Model file for the job. Use its own axes, mm. A direction names the side the tool comes from. Give positions to 0.01 mm unless a question says otherwise; leave off trailing zeros. Write each loop counter-clockwise with the first axis right and the second up, starting at its lowest first coordinate (ties: lowest second). Pieces come first, ordered by that corner, then holes.
```python
from build123d import *

# Parameters (mm, degrees)
SKETCH1_R            = 33.5
BOSS_EXTRUDE3_DEPTH  = 16.5
SKETCH2_W            = 20
SKETCH2_H            = 39
BOSS_EXTRUDE4_DEPTH  = 34.758
SKETCH3_R            = 10
SKETCH3_R_2          = 6.5
BOSS_EXTRUDE5_DEPTH  = 2
SKETCH3_3_R          = 6.5
BOSS_EXTRUDE6_DEPTH  = 3
SKETCH3_4_R          = 2.85
BOSS_EXTRUDE7_DEPTH  = 7.3
SKETCH5_W            = 11
SKETCH5_H            = 3.5
SKETCH5_W_2          = 3.5
SKETCH5_H_2          = 8
BOSS_EXTRUDE8_DEPTH  = 34.758
SKETCH6_W            = 11
SKETCH6_H            = 8
BOSS_EXTRUDE9_DEPTH  = 3.5
SKETCH7_R            = 2.5
BOSS_EXTRUDE10_DEPTH = 6
FILLET1_R            = 3.5
FILLET2_R            = 3.5
FILLET3_R            = 3.5
FILLET4_R            = 3.5
SKETCH9_W            = 3.5
SKETCH9_H            = 20
BOSS_EXTRUDE11_DEPTH = 30.867
SKETCH9_3_W          = 3.5
SKETCH9_3_H          = 11
BOSS_EXTRUDE12_DEPTH = 27
CUT_EXTRUDE1_DEPTH   = 88.052447203
BOSS_EXTRUDE13_START = 3
SKETCH10_3_R         = 10
BOSS_EXTRUDE13_DEPTH = 3
SKETCH10_4_R         = 5
SKETCH10_4_R_2       = 3
BOSS_EXTRUDE14_DEPTH = 4.5
CUT_EXTRUDE4_START   = -18.5
SKETCH10_7_R         = 1.5
CUT_EXTRUDE4_DEPTH   = 34.5
CIRPATTERN3_COUNT    = 4
SKETCH11_R           = 1.5
CUT_EXTRUDE6_DEPTH   = 86.054856205
SKETCH13_R           = 2.7
CUT_EXTRUDE10_DEPTH  = 15.5
CUT_EXTRUDE11_DEPTH  = 3.5
CIRPATTERN4_COUNT    = 4
SKETCH14_3_R         = 1.25
CUT_EXTRUDE12_DEPTH  = 3.5


with BuildPart() as part:
    # Sketch1 → Boss-Extrude3 (new body)
    with BuildSketch(Plane.XY):
        Circle(SKETCH1_R)
    extrude(amount=BOSS_EXTRUDE3_DEPTH)

    # Sketch2 → Boss-Extrude4 (add)
    with BuildSketch(Plane.XY.offset(16.5)):
        Rectangle(SKETCH2_W, SKETCH2_H)
    extrude(amount=BOSS_EXTRUDE4_DEPTH)

    # Sketch3 → Boss-Extrude5 (add)
    with BuildSketch(Plane(origin=(0, 19.5, 0), x_dir=(1, 0, 0), z_dir=(0, 1, 0))):
        with Locations(Location((0, -41.258, 0), (0, 0, 270))):
            Circle(SKETCH3_R)
        with Locations(Location((0, -41.258, 0), (0, 0, 270))):
            Circle(SKETCH3_R_2, mode=Mode.SUBTRACT)
    extrude(amount=BOSS_EXTRUDE5_DEPTH)

    # Sketch3<3> → Boss-Extrude6 (add)
    with BuildSketch(Plane(origin=(0, 19.5, 0), x_dir=(1, 0, 0), z_dir=(0, 1, 0))):
        with Locations(Location((0, -41.258, 0), (0, 0, 270))):
            Circle(SKETCH3_3_R)
    extrude(amount=BOSS_EXTRUDE6_DEPTH)

    # Sketch3<4> → Boss-Extrude7 (add)
    with BuildSketch(Plane(origin=(0, 19.5, 0), x_dir=(1, 0, 0), z_dir=(0, 1, 0))):
        with Locations(Location((0, -41.258, 0), (0, 0, 270))):
            Circle(SKETCH3_4_R)
    extrude(amount=BOSS_EXTRUDE7_DEPTH)

    # Sketch5 → Boss-Extrude8 (add)
    with BuildSketch(Plane.XY.offset(51.258)):
        with Locations((0, -21.25)):
            Rectangle(SKETCH5_W, SKETCH5_H)
        with Locations((11.75, 7.5)):
            Rectangle(SKETCH5_W_2, SKETCH5_H_2)
        with Locations((-11.75, 7.5)):
            Rectangle(SKETCH5_W_2, SKETCH5_H_2)
    extrude(amount=-BOSS_EXTRUDE8_DEPTH)

    # Sketch6 → Boss-Extrude9 (add)
    with BuildSketch(Plane.XY.offset(51.258)):
        with Locations((0, 7.5)):
            Rectangle(SKETCH6_W, SKETCH6_H)
        Polygon((10, 11.5), (5.5, 11.5), (5.5, 3.5), (10, 3.5), (13.5, 3.5), (13.5, 11.5), align=None)
        Polygon((5.5, 3.5), (-5.5, 3.5), (-5.5, -19.5), (-5.5, -23), (5.5, -23), (5.5, -19.5), align=None)
        Polygon((-10, 11.5), (-13.5, 11.5), (-13.5, 3.5), (-10, 3.5), (-5.5, 3.5), (-5.5, 11.5), align=None)
    extrude(amount=BOSS_EXTRUDE9_DEPTH)

    # Sketch7 → Boss-Extrude10 (add)
    with BuildSketch(Plane.XZ.offset(23)):
        with Locations(Location((0, 41.258, 0), (0, 0, 270))):
            Circle(SKETCH7_R)
    extrude(amount=BOSS_EXTRUDE10_DEPTH)

    # Fillet1
    fillet1_edges = [part.edges().sort_by_distance(p)[0] for p in [
        (-13.5, 7.5, 54.758),
        (13.5, 7.5, 54.758),
    ]]
    fillet(fillet1_edges, radius=FILLET1_R)

    # Fillet2
    fillet2_edges = [part.edges().sort_by_distance(p)[0] for p in [
        (0, -23, 54.758),
    ]]
    fillet(fillet2_edges, radius=FILLET2_R)

    # Fillet3
    fillet3_edges = [part.edges().sort_by_distance(p)[0] for p in [
        (13.5, 7.5, 16.5),
    ]]
    fillet(fillet3_edges, radius=FILLET3_R)

    # Fillet4
    fillet4_edges = [part.edges().sort_by_distance(p)[0] for p in [
        (-13.5, 7.5, 16.5),
    ]]
    fillet(fillet4_edges, radius=FILLET4_R)

    # Sketch9 → Boss-Extrude11 (add)
    with BuildSketch(Plane(origin=(0, 0, 0), x_dir=(-1, 0, 0), z_dir=(0, 0, -1))):
        with Locations((27.05, 0)):
            Rectangle(SKETCH9_W, SKETCH9_H)
    extrude(amount=BOSS_EXTRUDE11_DEPTH)

    # Sketch9<3> → Boss-Extrude12 (add)
    with BuildSketch(Plane(origin=(0, 0, 0), x_dir=(-1, 0, 0), z_dir=(0, 0, -1))):
        with Locations((-27.25, 0)):
            Rectangle(SKETCH9_3_W, SKETCH9_3_H)
    extrude(amount=BOSS_EXTRUDE12_DEPTH)

    # Sketch10 → Cut-Extrude1 (cut, through all)
    with BuildSketch(Plane(origin=(-25.3, 0, 0), x_dir=(0, 0, -1), z_dir=(1, 0, 0))):
        with BuildLine():
            ThreePointArc((20.867, 10), (27.938067812, 7.071067812), (30.867, 0))
            Line((30.867, 0), (30.867, 10))
            Line((30.867, 10), (20.867, 10))
        make_face()
        with BuildLine():
            Line((30.867, -10), (30.867, 0))
            ThreePointArc((30.867, 0), (27.938067812, -7.071067812), (20.867, -10))
            Line((20.867, -10), (30.867, -10))
        make_face()
    extrude(amount=-CUT_EXTRUDE1_DEPTH, mode=Mode.SUBTRACT)

    # Sketch10<3> → Boss-Extrude13 (add)
    with BuildSketch(Plane(origin=(-25.3, 0, 0), x_dir=(0, 0, -1), z_dir=(1, 0, 0)).offset(BOSS_EXTRUDE13_START)):
        with Locations(Location((20.867, 0, 0), (0, 0, 90))):
            Circle(SKETCH10_3_R)
    extrude(amount=-BOSS_EXTRUDE13_DEPTH)

    # Sketch10<4> → Boss-Extrude14 (add)
    with BuildSketch(Plane(origin=(-25.3, 0, 0), x_dir=(0, 0, -1), z_dir=(1, 0, 0))):
        with Locations(Location((20.867, 0, 0), (0, 0, 90))):
            Circle(SKETCH10_4_R)
        with Locations(Location((20.867, 0, 0), (0, 0, 90))):
            Circle(SKETCH10_4_R_2, mode=Mode.SUBTRACT)
    extrude(amount=BOSS_EXTRUDE14_DEPTH)

    # Sketch10<7> → Cut-Extrude4 (cut)
    with BuildSketch(Plane(origin=(-25.3, 0, 0), x_dir=(0, 0, -1), z_dir=(1, 0, 0)).offset(CUT_EXTRUDE4_START)):
        with Locations(Location((20.867, -7, 0), (0, 0, 180))):
            Circle(SKETCH10_7_R)
    cut_extrude4 = extrude(amount=CUT_EXTRUDE4_DEPTH, mode=Mode.SUBTRACT)

    # CirPattern3: Cut-Extrude4 ×4 about axis
    cirpattern3_axis = Axis((0, 0, -20.867), (1, 0, 0))
    for i in range(1, CIRPATTERN3_COUNT):
        add(cut_extrude4.rotate(cirpattern3_axis, i * 360 / CIRPATTERN3_COUNT), mode=Mode.SUBTRACT)

    # Sketch11 → Cut-Extrude6 (cut, through all)
    with BuildSketch(Plane(origin=(-22.3, 0, 0), x_dir=(0, 0, -1), z_dir=(1, 0, 0))):
        with Locations(Location((20.867, 0, 0), (0, 0, 90))):
            Circle(SKETCH11_R)
    extrude(amount=-CUT_EXTRUDE6_DEPTH, mode=Mode.SUBTRACT)

    # Sketch13 → Cut-Extrude10 (cut)
    with BuildSketch(Plane(origin=(29, 0, 0), x_dir=(0, 0, -1), z_dir=(1, 0, 0))):
        with BuildLine():
            ThreePointArc((20.867, 5.5), (24.756087297, 3.889087297), (26.367, 0))
            ThreePointArc((26.367, 0), (24.756087297, -3.889087297), (20.867, -5.5))
            Line((20.867, -5.5), (27, -5.5))
            Line((27, -5.5), (27, 5.5))
            Line((27, 5.5), (20.867, 5.5))
        make_face()
        with Locations((20.867, 0)):
            Circle(SKETCH13_R)
    extrude(amount=-CUT_EXTRUDE10_DEPTH, mode=Mode.SUBTRACT)

    # Sketch14 → Cut-Extrude11 (cut)
    with BuildSketch(Plane(origin=(0, 0, 0), x_dir=(-1, 0, 0), z_dir=(0, 0, -1))):
        with BuildLine():
            Line((0, 18), (0, 9))
            ThreePointArc((0, 9), (2.329371406, 8.693332437), (4.5, 7.794228634))
            Line((4.5, 7.794228634), (9, 15.588457268))
            ThreePointArc((9, 15.588457268), (4.658742812, 17.386664873), (0, 18))
        make_face()
        with BuildLine():
            ThreePointArc((-4.5, 7.794228634), (-2.329371406, 8.693332437), (0, 9))
            Line((0, 9), (0, 18))
            ThreePointArc((0, 18), (-4.658742812, 17.386664873), (-9, 15.588457268))
            Line((-9, 15.588457268), (-4.5, 7.794228634))
        make_face()
    cut_extrude11 = extrude(amount=-CUT_EXTRUDE11_DEPTH, mode=Mode.SUBTRACT)

    # CirPattern4: Cut-Extrude11 ×4 about axis
    cirpattern4_axis = Axis((0, 0, 0), (0, 0, 1))
    for i in range(1, CIRPATTERN4_COUNT):
        add(cut_extrude11.rotate(cirpattern4_axis, i * 360 / CIRPATTERN4_COUNT), mode=Mode.SUBTRACT)

    # Sketch14<3> → Cut-Extrude12 (cut)
    with BuildSketch(Plane(origin=(0, 0, 0), x_dir=(-1, 0, 0), z_dir=(0, 0, -1))):
        Circle(SKETCH14_3_R)
    extrude(amount=-CUT_EXTRUDE12_DEPTH, mode=Mode.SUBTRACT)


solid = part.part
```
1. Slice it at D-D, the plane z = 13. Write the cut outline in (x, y), and give its area (3 significant figures).
Calculated:
outline: circle Ø67 at (0, 0)
area: 3,530 mm2
2. Slice it at B-B, the plane x = -24. Write the cut outline in (y, z).
Calculated:
outline: (-23.37, 0) - (23.37, 0) - (23.37, 16.5) - (-23.37, 16.5) - close; circle Ø20 at (0, -20.87); hole circle Ø3 at (-7, -20.87); hole circle Ø3 at (0, -27.87); hole circle Ø3 at (0, -20.87); hole circle Ø3 at (0, -13.87); hole circle Ø3 at (7, -20.87)
3. Pin check, flat tips, straight feed: P1, Ø6, axis at x = 21, z = 11, coming from the +Y side; P2, Ø1.5, axis at x = -23, y = 24.5, coming from the -Z side; P3, Ø4, axis at y = 7, z = -20.867, coming from the +X side. Stop position of each tip, or through.
Calculated:
P1: stops at y = 28.25
P2: stops at z = 0
P3: stops at x = 29
4. Pull direction Y, two halves, no side cores. Call faces 4 (the flat face through (5.5, -20, 40)), 5 (the flat face through (0, 13, 3.5)), 6 (the flat face through (0, 19.5, 26)), 7 (the flat face through (27, -5.5, -10)): +Y half, -Y half, draft (parallel to the pull), parting line (faces both ways), or undercut.
Calculated:
face 4: draft
face 5: undercut
face 6: +Y half
face 7: -Y half
5. Slice it at C-C, the plane z = 29. Write the cut outline in (x, y), and give its area (4 significant figures).
Calculated:
outline: (-13.5, 3.5) - (-10, 3.5) - (-10, -19.5) - (-5.5, -19.5) - (-5.5, -23) - (5.5, -23) - (5.5, -19.5) - (10, -19.5) - (10, 3.5) - (13.5, 3.5) - (13.5, 11.5) - (10, 11.5) - (10, 19.5) - (-10, 19.5) - (-10, 11.5) - (-13.5, 11.5) - close
area: 874.5 mm2
6. Probe probe 1 along X at (y, z) = (3, -12); probe 2 along X at (y, z) = (0.5, -8.5); probe 3 along Z at (x, y) = (12.5, -5.5). List the from-to ranges inside material, lowest first.
Calculated:
probe 1: x = -28.8 to -22.3, 25.5 to 29
probe 2: x = -28.8 to -25.3, 25.5 to 29
probe 3: z = 3.5 to 16.5
7. Slice it at A-A, the plane z = -6. Write the cut outline in (x, y), and give its area (4 significant figures).
Calculated:
outline: (-28.8, -10) - (-25.3, -10) - (-25.3, 10) - (-28.8, 10) - close; (25.5, -5.5) - (29, -5.5) - (29, 5.5) - (25.5, 5.5) - close
area: 108.5 mm2
8. Which spindle directions (+Z, -Z, +X, -X, +Y, -Y) get a long thin tool onto all of the face, cutting with end or side? Do faces 1 (the flat face through (-10, 15, 34)), 2 (the flat face through (-11.746, 6.782, 1.726)), 3 (the flat face through (13.5, 7, 35)). Say none if no direction does.
Calculated:
face 1: +Z, -X, +Y
face 2: -Z
face 3: +Z, +X, +Y, -Y
